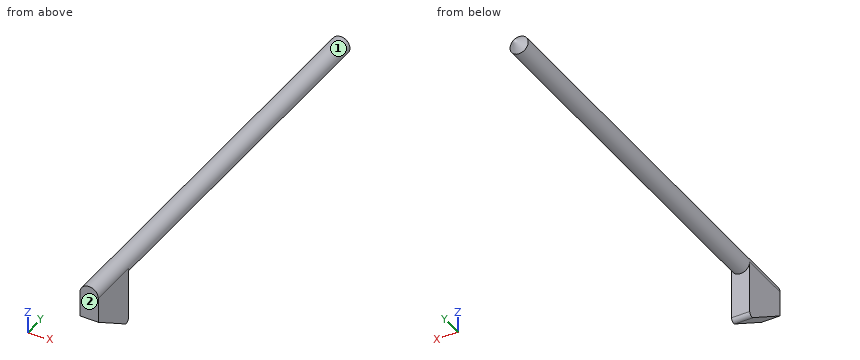
```python
from build123d import *

# Parameters (mm, degrees)
F0_R        = 2.5
F1_DEPTH    = 105
F3_DEPTH    = 14
F4_SIZE     = 2.5
F5_T1_DEPTH = 82.5140157162
F6_R        = 1


# Not quite as in the source:
# - a fillet or chamfer that OpenCascade refuses, or shapes differently, is made with other operations: its cross-section is extruded or revolved along the edge and cut away or added


with BuildPart() as f1:
    # F0 (on Front) → F1 (new body)
    with BuildSketch(Plane.XZ):
        Circle(F0_R)
    extrude(amount=-F1_DEPTH)

    # F2 (on face) → F3 (join)
    with BuildSketch(Plane.XZ):
        with BuildLine():
            Line((-2.5, 0), (-2.5, -17))
            Line((-2.5, -17), (2.5, -17))
            Line((2.5, -17), (2.5, 0))
            ThreePointArc((2.5, 0), (0, -2.5), (-2.5, 0))
        make_face()
        with BuildLine():
            ThreePointArc((2.5, 0), (0, 2.5), (-2.5, 0))
            ThreePointArc((-2.5, 0), (0, -2.5), (2.5, 0))
        make_face()
    extrude(amount=F3_DEPTH)

    # F4
    f4_edges = [f1.edges().sort_by_distance(p)[0] for p in [
        (-2.5, 105, 0),
    ]]
    chamfer(f4_edges, length=F4_SIZE)

    # F5: chamfer of 10 x 15 on 1 edges, made by hand

    # F5_s2 → F5_t1 (cut)
    with BuildSketch(Plane.YZ.offset(-41.2570078581)):
        Polygon((-14, -7), (1, -17), (-14, -17), align=None)
    extrude(amount=F5_T1_DEPTH, mode=Mode.SUBTRACT)

    # F6
    f6_edges = [f1.edges().sort_by_distance(p)[0] for p in [
        (0, 0, -16.333333),
    ]]
    fillet(f6_edges, radius=F6_R)


solid = f1.part
```
Can you work these out from the model? Positions are in its coordinate system, mm. Face numbers are marked on the shaded views. A direction names the side the tool comes from. Coordinates: 2 decimals unless noted, no trailing zeros. Loops run counter-clockwise (first coordinate to the right, second up) from the corner with the lowest first, then second, coordinate; pieces in that order, holes last. Notation, with made-up numbers: (-6, 74.25) - (30, 74.25) arc R25 cw to (30, 94.25) - close; hole circle Ø9 at (68.5, 23.5). An arc over 180 degrees is marked (long way). Use a Markdown table: item, result.
Item 1: I want a section at A-A on z = -3.5. Please give me the cut outline in (x, y), and give its area (3 significant figures).
Numbers:
| item | result |
|---|---|
| outline | (-2.5, -14) - (2.5, -14) - (2.5, 0) - (-2.5, 0) - close |
| area | 70.0 mm2 |
Item 2: I want a section at C-C on z = -9.5. Please give me the cut outline in (x, y).
Numbers:
| item | result |
|---|---|
| outline | (-2.5, -10.25) - (2.5, -10.25) - (2.5, 0) - (-2.5, 0) - close |
Item 3: If I drill on probe 1 along Z at (x, y) = (0.15, 49); probe 2 along Y at (x, z) = (-1.15, -4.5); probe 3 along Z at (x, y) = (-1.65, 56), over which ranges is the centre line in solid material (lowest first)? Write a range as from..to.
Numbers:
| item | result |
|---|---|
| probe 1 | z = -2.5..2.5 |
| probe 2 | y = -14..0 |
| probe 3 | z = -1.88..1.88 |
Item 4: For the marked faces 1 and 2, which set-ups out of +Z, -Z, +X, -X, +Y, -Y let a thin tool reach every point of the face, with its end or its side?
Numbers:
| item | result |
|---|---|
| face 1 | +Y |
| face 2 | +Z, -Z, +X, -X, -Y |
Item 5: I want a section at B-B on y = 45. Please give me the cut outline in (x, z).
Numbers:
| item | result |
|---|---|
| outline | circle Ø5 at (0, 0) |
Item 6: Will this pin go through, and if not, where does the flat tip stop? pin 1 (2.5 mm diameter, centred on x = 0.5, z = -8, fed in from +Y).
Numbers:
| item | result |
|---|---|
| pin 1 | stops at y = 0 |
